Verification items for the finished model (mm, model axes). A direction names the side the tool comes from. Coordinates: 2 decimals unless noted, no trailing zeros. Order: outer loops, then holes, each group sorted by start corner. A loop starts at its lowest first (then second) coordinate and runs counter-clockwise, first axis right, second up. Notation, with made-up numbers: M -21,-12.75 L -8,-12.75 A25 ccw -8,24.25 Z; hole C 55,81.5 d8. An arc over 180 degrees is marked long. Return JSON: item names as keys, results as strings. Group by question number.
Q1. Access from +Z, -Z, +X, -X, +Y, -Y to the whole of each face (thin tool, end or side, straight path). Record for faces 1 (the face through (0, -4.65, 4)), 2 (the face through (47.5, 1, 5)), 3 (the face through (-3.5, 3, 9)), 4 (the face through (-1, -7, 10.049)).
Q2. Mould release check, pull along Y, two halves, no side actions. Record for faces 5 (the face through (-1, -11.48, 13)), 6 (the face through (0, 0, 9)), 7 (the face through (-1, -2, 18)), 8 (the face through (25, 1.6, 9.1)): pulls with the +Y half, pulls with the -Y half, needs draft (parallel to the pull), parting line crosses it, or undercut.
Q3. Section check B-B, the plane z = 3.5. Enter the section's corners in (x, y), then the cut area to 3 significant figures.
Q4. Thickness scan on probe 1 along Y at (x, z) = (23.5, 13.5); probe 2 along Y at (x, z) = (-23.5, 4.5); probe 3 along X at (y, z) = (-2.5, 5.75). Record the ranges inside material, lowest first.
Q5. Go/stop test with flat-tipped pins: pin 1 Ø3 at (y, z) = (1, 5.5) entering from +X; pin 2 Ø3.5 at (x, z) = (0, 6.5) entering from +Y; pin 3 Ø6.5 at (x, z) = (20.5, 2.5) entering from -Y. Record where each tip stops, or that it passes through.
Q6. Section check A-A, the plane x = -23.5. Enter the section's corners in (y, z).
from build123d import *

# Parameters (mm, degrees)
BOSS_EXTRU_1_DEPTH      = 18
ESQUISSE2_R             = 1.5
ENL_V_MAT_EXTRU_1_DEPTH = 52.008553204
ESQUISSE3_W             = 7.950993182
ESQUISSE3_H             = 6.830138408
BOSS_EXTRU_2_DEPTH      = 95
ESQUISSE4_W             = 20
ESQUISSE4_H             = 16.130138408
BOSS_EXTRU_3_DEPTH      = 7.950993182
CONG_1_R                = 2


with BuildPart() as part:
    # Esquisse1 → Boss.-Extru.1 (new body)
    with BuildSketch(Plane.XY):
        Polygon((-47.5, 4.65), (-3.5, 4.65), (-3.5, 0), (3.5, 0), (3.5, 4.65), (47.5, 4.65), (47.5, -4.65), (-47.5, -4.65), align=None)
    extrude(amount=BOSS_EXTRU_1_DEPTH)

    # Esquisse2 → Enlèv. mat.-Extru.1 (cut, through all)
    with BuildSketch(Plane.XY.offset(18)):
        with Locations((-23.5, 1.65)):
            Circle(ESQUISSE2_R)
        with Locations(Location((23.5, 1.65, 0), (0, 0, 180))):
            Circle(ESQUISSE2_R)
    extrude(amount=-ENL_V_MAT_EXTRU_1_DEPTH, mode=Mode.SUBTRACT)

    # Esquisse3 → Boss.-Extru.2 (add)
    with BuildSketch(Plane.ZY.offset(47.5)):
        with Locations((14.024503409, -8.065069204)):
            Rectangle(ESQUISSE3_W, ESQUISSE3_H)
    extrude(amount=-BOSS_EXTRU_2_DEPTH)

    # Esquisse4 → Boss.-Extru.3 (add)
    with BuildSketch(Plane.XY.offset(18)):
        with Locations((-57.5, -3.415069204)):
            Rectangle(ESQUISSE4_W, ESQUISSE4_H)
        with Locations((57.5, -3.415069204)):
            Rectangle(ESQUISSE4_W, ESQUISSE4_H)
    extrude(amount=-BOSS_EXTRU_3_DEPTH)

    # Congé1
    cong_1_edges = [part.edges().sort_by_distance(p)[0] for p in [
        (-47.5, 4.65, 5.024503409),
        (0, -4.65, 10.049006818),
        (0, -11.480138408, 18),
        (-3.5, 0, 9),
        (3.5, 0, 9),
        (-57.5, 4.65, 10.049006818),
        (47.5, -4.65, 5.024503409),
        (47.5, 0, 0),
        (-47.5, 0, 0),
        (47.5, 0, 10.049006818),
        (-47.5, 0, 10.049006818),
        (67.5, 4.65, 14.024503409),
        (67.5, -11.480138408, 14.024503409),
        (-67.5, 4.65, 14.024503409),
        (-67.5, -11.480138408, 14.024503409),
    ]]
    fillet(cong_1_edges, radius=CONG_1_R)


solid = part.part
Numbers:
{
 "1": {"face 1": "-Z, +X, -X, -Y", "face 2": "-Z, +X, +Y, -Y", "face 3": "+Z, -Z, +Y", "face 4": "-Z, -Y"},
 "2": {"face 5": "pulls with the -Y half", "face 6": "pulls with the +Y half", "face 7": "needs draft", "face 8": "undercut"},
 "3": {"outline": "M -47.5,-4.65 L 45.5,-4.65 A2 ccw 47.5,-2.65 L 47.5,4.65 L 3.5,4.65 L 3.5,2 A2 cw 1.5,0 L -1.5,0 A2 cw -3.5,2 L -3.5,4.65 L -45.5,4.65 A2 ccw -47.5,2.65 Z; hole C -23.5,1.65 d3; hole C 23.5,1.65 d3", "area": "837 mm2"},
 "4": {"probe 1": "y = -11.48 to 0.15, 3.15 to 4.65", "probe 2": "y = -4.65 to 0.15, 3.15 to 4.65", "probe 3": "x = -47.5 to 47.5"},
 "5": {"pin 1": "stops at x = 47.5", "pin 2": "stops at y = 0.02", "pin 3": "stops at y = -4.65"},
 "6": {"outline": "M -11.48,10.05 L -6.65,10.05 A2 cw -4.65,8.05 L -4.65,0 L 0.15,0 L 0.15,18 L -9.48,18 A2 ccw -11.48,16 Z; M 3.15,0 L 4.65,0 L 4.65,18 L 3.15,18 Z"}
}
